Source: three-view drawing plus pictorial views. Frame: mm from the lowest corner of the part. Give positions to 0.01 mm unless a question says otherwise; leave off trailing zeros. Order: outer loops, then holes, each group sorted by start corner. A loop starts at its lowest first (then second) coordinate and runs counter-clockwise, first axis right, second up. Notation, with made-up numbers: (22, 21) - (54, 21) arc R28 ccw to (54, 52) - close; hole circle Ø10 at (-22.75, -13). An arc over 180 degrees is marked (long way). Use one line per item in the form item = value.
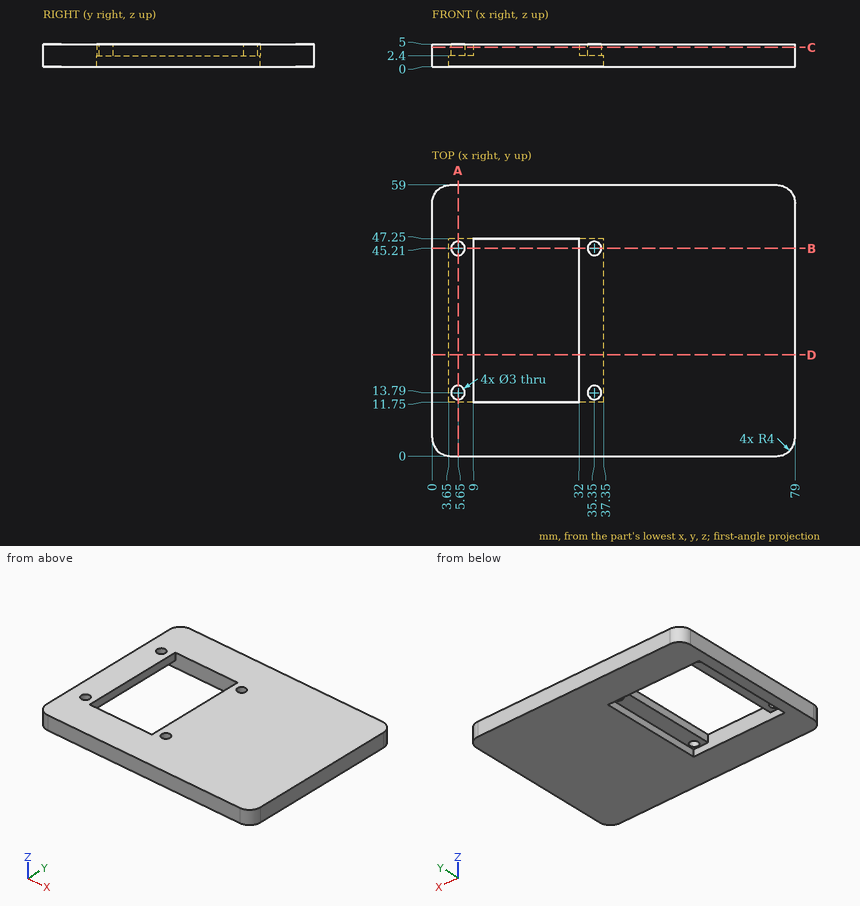
(1) Cut plane D-D on y = 22. Output: boundary loops of the cut face in (x, z).
Computed values:
outline = (0, 0) - (3.65, 0) - (3.65, 2.4) - (9, 2.4) - (9, 5) - (0, 5) - close; (32, 2.4) - (37.35, 2.4) - (37.35, 0) - (79, 0) - (79, 5) - (32, 5) - close
(2) Ray query, line 1 along Y through (x, z) = (5.5, 3.2); line 2 along X through (y, z) = (36, 2); line 3 along Y through (x, z) = (36.5, 1.85). Return the intervals inside material, ascending.
Computed values:
line_1 = 0 to 12.3, 15.28 to 43.72, 46.7 to 59
line_2 = 0 to 3.65, 37.35 to 79
line_3 = 0 to 11.75, 47.25 to 59
(3) Cut plane A-A on x = 5.65. Output: boundary loops of the cut face in (y, z), plus the area to 3 significant figures.
Computed values:
outline = (0, 0) - (11.75, 0) - (11.75, 2.4) - (12.29, 2.4) - (12.29, 5) - (0, 5) - close; (15.29, 2.4) - (43.71, 2.4) - (43.71, 5) - (15.29, 5) - close; (46.71, 2.4) - (47.25, 2.4) - (47.25, 0) - (59, 0) - (59, 5) - (46.71, 5) - close
area = 194 mm²
(4) Cut plane C-C on z = 4.25. Output: boundary loops of the cut face in (x, y), plus the area to 3 significant figures.
Computed values:
outline = (0, 4) arc R4 ccw to (4, 0) - (75, 0) arc R4 ccw to (79, 4) - (79, 55) arc R4 ccw to (75, 59) - (4, 59) arc R4 ccw to (0, 55) - close; hole circle Ø3 at (5.65, 13.79); hole circle Ø3 at (5.65, 45.21); hole (9, 11.75) - (32, 11.75) - (32, 47.25) - (9, 47.25) - close; hole circle Ø3 at (35.35, 13.79); hole circle Ø3 at (35.35, 45.21)
area = 3,800 mm²
(5) Contact query for flat-ended pins moving along their axis: pin 1 Ø2.5 at (x, y) = (5.65, 13.79) entering from -Z; pin 2 Ø3.5 at (x, y) = (5.65, 45.21) entering from -Z; pin 3 Ø0.7 at (y, z) = (24.5, 1) entering from -X. Output: stop coordinate, or through.
Computed values:
pin_1 = through
pin_2 = 2.4
pin_3 = 0
(6) Cut plane B-B on y = 45.21. Output: boundary loops of the cut face in (x, z), plus the area to 3 significant figures.
Computed values:
outline = (0, 0) - (3.65, 0) - (3.65, 2.4) - (4.15, 2.4) - (4.15, 5) - (0, 5) - close; (7.15, 2.4) - (9, 2.4) - (9, 5) - (7.15, 5) - close; (32, 2.4) - (33.85, 2.4) - (33.85, 5) - (32, 5) - close; (36.85, 2.4) - (37.35, 2.4) - (37.35, 0) - (79, 0) - (79, 5) - (36.85, 5) - close
area = 239 mm²
